Can you work these out from the drawing? Everything is in mm from the part's minimum corner. Round coordinates to 2 decimals unless told otherwise and drop trailing zeros. Loops run counter-clockwise (first coordinate to the right, second up) from the corner with the lowest first, then second, coordinate; pieces in that order, holes last. Notation, with made-up numbers: (-35, 64.25) - (23, 64.25) arc R25 cw to (23, 77.25) - close; hole circle Ø6 at (-10, 50). An arc over 180 degrees is marked (long way). Return JSON: item names as keys, results as strings. Group by question number.
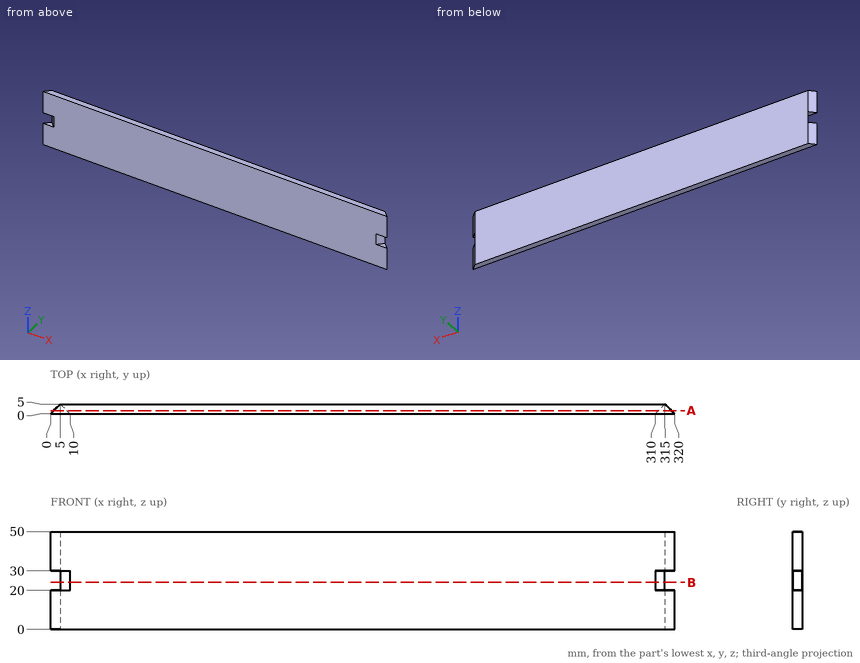
Q1. Imagine slicing it at A-A, the plane y = 1.6. List the corners of the cut face in (x, z) for me, and give its area (3 significant figures).
Q2. Imagine slicing it at B-B, the plane z = 24. List the corners of the cut face in (x, y) for me.
Q3. Will these pins go through, and if not, where does the flat tip stop? pin 1 Ø1.5 at (y, z) = (3, 29.5) entering from -X; pin 2 Ø2 at (y, z) = (3, 22) entering from +X.
Q4. Please list where these lines run through material, in increasing order: line 1 (X direction, y = 4.3, z = 15.5); line 2 (X direction, y = 1.85, z = 31).
Output values:
{
 "1": {"outline": "(1.6, 0) - (318.4, 0) - (318.4, 20) - (311.6, 20) - (311.6, 30) - (318.4, 30) - (318.4, 50) - (1.6, 50) - (1.6, 30) - (8.4, 30) - (8.4, 20) - (1.6, 20) - close", "area": "15,700 mm^2"},
 "2": {"outline": "(5, 5) - (10, 0) - (310, 0) - (315, 5) - close"},
 "3": {"pin 1": "stops at x = 2.44", "pin 2": "stops at x = 314"},
 "4": {"line 1": "x = 4.3 to 315.7", "line 2": "x = 1.85 to 318.15"}
}
